from build123d import *

# Parameters (mm, degrees)
SKETCH1_R                  = 3
BOSS_EXTRUDE1_DEPTH        = 15
SHAFT_START                = -15
SHAFT_D_DEPTH              = 15
CUT_EXTRUDE1_DEPTH         = 66.3834841531101
BOSS_EXTRUDE3_DEPTH        = 0.9
CUT_EXTRUDE2_DEPTH         = 59.56795722653927
SHAFT_HOLE_EXPANSION_DEPTH = 59.56795722653927
CUT_EXTRUDE4_DEPTH         = 59.56795722653927
FILLET1_R                  = 2


with BuildPart() as part:
    # Sketch1 → Boss-Extrude1 (new body)
    with BuildSketch(Plane(origin=(0, 0, 0), x_dir=(1, 0, 0), z_dir=(0, 1, 0))):
        with BuildLine():
            Line((-31.81980515339447, 31.819805153394796), (-7.071067811865444, 7.071067811865506))
            ThreePointArc((-7.071067811865444, 7.071067811865506), (4.724e-14, 10.000000000000002), (7.071067811865511, 7.071067811865442))
            Line((7.071067811865511, 7.071067811865442), (31.819805153394796, 31.819805153394476))
            ThreePointArc((31.819805153394796, 31.819805153394476), (-2.4807e-13, -44.99999999999999), (-31.81980515339447, 31.819805153394796))
        make_face()
        with Locations(Location((0, 0, 0), (0, 0, 270))):
            Circle(SKETCH1_R, mode=Mode.SUBTRACT)
    extrude(amount=BOSS_EXTRUDE1_DEPTH)

    # Sketch2 → Shaft D (add)
    with BuildSketch(Plane(origin=(0, 15, 0), x_dir=(1, 0, 0), z_dir=(0, 1, 0)).offset(SHAFT_START)):
        with BuildLine():
            Line((2.499999999999999, 1.6583123951777017), (2.499999999999999, -1.6583123951777017))
            ThreePointArc((2.499999999999999, -1.6583123951777017), (3.0000000000000004, 0), (2.499999999999999, 1.6583123951777017))
        make_face()
    extrude(amount=SHAFT_D_DEPTH)

    # Sketch4 → Cut-Extrude1 (cut, through all)
    with BuildSketch(Plane(origin=(0, 15, 0), x_dir=(1, 0, 0), z_dir=(0, 1, 0))):
        with BuildLine():
            Line((11.490666646784653, -9.641814145298108), (45.50378986806941, 30.893447649017453))
            ThreePointArc((45.50378986806941, 30.893447649017453), (34.99275019793601, -42.43238661193652), (-38.99293957205545, -38.78853778540811))
            Line((-38.99293957205545, -38.78853778540811), (11.490666646784653, -9.641814145298108))
        make_face()
    extrude(amount=-CUT_EXTRUDE1_DEPTH, mode=Mode.SUBTRACT)

    # Sketch6 → Boss-Extrude3 (add)
    with BuildSketch(Plane(origin=(7.0476946558942295, 0, 12.206965220240622), x_dir=(0.8660254037844414, 0, -0.4999999999999952), z_dir=(0.4999999999999952, 0, 0.8660254037844414))):
        Polygon((-42.73546536717619, 15), (5.130302149885087, 15), (5.130302149885089, 0), (-42.73546536717619, 0), align=None)
    extrude(amount=BOSS_EXTRUDE3_DEPTH)

    # Sketch7 → Cut-Extrude2 (cut, through all)
    with BuildSketch(Plane(origin=(0, 15, 0), x_dir=(1, 0, 0), z_dir=(0, 1, 0))):
        with BuildLine():
            Line((-31.525106333140414, 17.38297070940953), (-7.071067811865441, -7.07106781186544))
            Line((-7.071067811865441, -7.07106781186544), (-29.802141727564482, -20.19485945606356))
            ThreePointArc((-29.802141727564482, -20.19485945606356), (-35.962218628181056, -1.6488879097460596), (-31.525106333140414, 17.38297070940953))
        make_face()
    extrude(amount=-CUT_EXTRUDE2_DEPTH, mode=Mode.SUBTRACT)

    # Sketch9 → Shaft Hole Expansion (cut, through all)
    with BuildSketch(Plane(origin=(0, 15, 0), x_dir=(1, 0, 0), z_dir=(0, 1, 0))):
        with BuildLine():
            Line((2.5899999999999985, 1.685229954635274), (2.5899999999999985, -1.6852299546352736))
            ThreePointArc((2.5899999999999985, -1.6852299546352736), (-3.09, 3.8e-16), (2.5899999999999985, 1.685229954635274))
        make_face()
    extrude(amount=-SHAFT_HOLE_EXPANSION_DEPTH, mode=Mode.SUBTRACT)

    # Sketch10 → Cut-Extrude4 (cut, through all)
    with BuildSketch(Plane(origin=(0, 15, 0), x_dir=(1, 0, 0), z_dir=(0, 1, 0))):
        Polygon((11.49066664678465, -9.641814145298104), (7.493411323151681, -14.405557537754012), (21.666837443070385, -15.28946640390601), align=None)
    extrude(amount=-CUT_EXTRUDE4_DEPTH, mode=Mode.SUBTRACT)

    # Fillet1
    # the kernel refuses this fillet: 2 mm, written as the material it adds along each edge
    with BuildSketch(Plane(origin=(-29.802141727564482, 15, 20.19485945606356), x_dir=(0.8660254037844384, 0, -0.5000000000000004), z_dir=(0, -1, 0))) as fillet1_piece_1:
        with BuildLine():
            CenterArc((1.9119296968147805, -2.000000000000001), FILLET1_R, 90.00000000000006, 89.00874965826159)
            ThreePointArc((-0.08777100050710222, -1.9654005617043746), (-0.05731387291771985, -0.9821005956140282), (0, 0))
            Line((0, 0), (1.911929696814779, 4e-17))
        make_face()
    extrude(amount=15)
    with BuildSketch(Plane(origin=(-31.525106333140414, 15, -17.382970709409527), x_dir=(-0.44779859611608247, 0, 0.8941344514760997), z_dir=(0, -1, 0))) as fillet1_piece_2:
        with BuildLine():
            CenterArc((2.77241732034655, -1.9984307521616007), FILLET1_R, 87.73015185982399, 110.66731649351249)
            Line((0.8746374046450249, -2.6296449721851296), (0, 0))
            ThreePointArc((0, 0), (1.4258146218925176, 0.02824646109120102), (2.8516292437850255, 6e-17))
        make_face()
    extrude(amount=15)
    with BuildSketch(Plane(origin=(-7.071067811865441, 15, 7.07106781186544), x_dir=(-0.8660254037844387, 0, 0.4999999999999999), z_dir=(0, -1, 0))) as fillet1_piece_3:
        with BuildLine():
            CenterArc((FILLET1_R * 1.30322537284, FILLET1_R), FILLET1_R, 165.00000000000003, 104.99999999999997)
            Line((FILLET1_R * 0.337299546552, FILLET1_R * 1.2588190451), (0, 0))
            Line((0, 0), (FILLET1_R * 1.30322537284, 1e-17))
        make_face()
    extrude(amount=15)
    with BuildSketch(Plane(origin=(-7.071067811865445, 0, -7.071067811865506), x_dir=(-0.7071067811865437, 0, -0.7071067811865515), z_dir=(0, 1, 0))) as fillet1_piece_4:
        with BuildLine():
            CenterArc((1.8321595661992367, -2), FILLET1_R, 89.99999999999999, 80.40593177313956)
            ThreePointArc((-0.13986702816730157, -1.666666666666667), (-0.0350281054503974, -0.8362626027968331), (0, 0))
            Line((0, 0), (1.8321595661992371, 5e-17))
        make_face()
    extrude(amount=15)
    with BuildSketch(Plane(origin=(7.071067811865512, 0, -7.071067811865442), x_dir=(0.7071067811865507, 0, -0.7071067811865444), z_dir=(0, 1, 0))) as fillet1_piece_5:
        with BuildLine():
            CenterArc((1.8321595661992343, 2.0000000000000004), FILLET1_R, 189.59406822686037, 80.40593177313957)
            ThreePointArc((-0.139867028167305, 1.6666666666666698), (-0.03502810545039883, 0.8362626027968333), (0, 0))
            Line((0, 0), (1.8321595661992325, 4e-17))
        make_face()
    extrude(amount=15)
    # the kernel refuses this fillet: 2 mm, written as the material it takes off along each edge
    with BuildSketch(Plane(origin=(-29.512303994630546, -4.175823272127531, 34.35412076723451), x_dir=(-0.49999999999865496, 0, -0.8660254037852152), z_dir=(0, 1, 0))) as fillet1_2_piece_1:
        with BuildLine():
            CenterArc((2.0000000000025833, -1.6703293088479174), FILLET1_R, 123.36701296928852, 56.63298703080011)
            Line((2.58454e-12, -1.6703293088510118), (0, 0))
            Line((0, 0), (0.9000000000009275, 2e-17))
        make_face()
    extrude(amount=23.35164654425506, mode=Mode.SUBTRACT)
    with BuildSketch(Plane(origin=(9.799219929370043, -0.8816349035423467, 11.657601847458647), x_dir=(0.6427876096865316, 0, -0.7660444431189845), z_dir=(0, 1, 0))) as fillet1_2_piece_2:
        with BuildLine():
            CenterArc((FILLET1_R * 0.176326980708, FILLET1_R), FILLET1_R, 249.99999999999906, 20.000000000000284)
            Line((-FILLET1_R * 0.165693162617, FILLET1_R * 0.0603073792141), (0, 0))
            Line((0, 0), (FILLET1_R * 0.176326980708, 1e-17))
        make_face()
    extrude(amount=16.763269807084693, mode=Mode.SUBTRACT)
    with BuildSketch(Plane(origin=(38.76183530710732, 18.67919870008775, -22.858699079883973), x_dir=(-0.5219883581091025, 0, -0.8529526094681715), z_dir=(0, -1, 0))) as fillet1_2_piece_3:
        with BuildLine():
            CenterArc((1.4389754915898811, -1.9997325944085071), FILLET1_R, 89.06305798679442, 72.40266339187922)
            Line((-0.45729180864609936, -1.363988678939587), (0, 0))
            ThreePointArc((0, 0), (0.7358397400175548, 0.00601662580861232), (1.4716794800350999, 0))
        make_face()
    extrude(amount=22.3583974001755, mode=Mode.SUBTRACT)


solid = part.part
Check sheet for the modelled part. Datum: model origin and axes. Units: mm. A direction names the side the tool comes from. Round coordinates to 2 decimals unless told otherwise and drop trailing zeros. Write each loop counter-clockwise with the first axis right and the second up, starting at its lowest first coordinate (ties: lowest second). Pieces come first, ordered by that corner, then holes. Notation, with made-up numbers: (-7.75, 76.5) -> (9.25, 76.5) arc R9 ccw to (9.25, 92.5) -> close; hole circle Ø6 at (-21.5, 0). An arc over 180 degrees is marked (long way). Answer as CSV lines item,"result". Start each with the question number.
1) Tool access check on faces 1 (the flat face through (-20, 7, -20)), 2 (the cylindrical face through (38.3, 7.6, -22.9)), 3 (the cylindrical face through (-29.626, 7.605, 19.448)). Record the directions out of +Z, -Z, +X, -X, +Y, -Y that give a thin tool (end or side, any length) a straight path to the whole face; none if there is none.
2) Release check for a two-part mould opening along Z. For faces 4 (the cylindrical face through (-29.021, 7.395, 33.786)), 5 (the flat face through (-18.606, 7.605, 13.731)), 6 (the cylindrical face through (35.075, 7.395, -28.191)) record: pulls with the +Z half, pulls with the -Z half, needs draft (parallel to the pull), parting line crosses it, or undercut.
3) Section check B-B on z = 0. Enter the section's corners in (x, y), and give its area (3 significant figures).
4) Section check A-A on y = 5.25. Enter the section's corners in (x, z), and give its area (3 significant figures).
5) Go/stop test with flat-tipped pins: P1, Ø6, axis at y = 7.5, z = 25.5, coming from the +X side; P2, Ø8, axis at y = 2, z = 19.5, coming from the +X side; P3, Ø4, axis at x = -2.5, y = 4.5, coming from the -Z side; P4, Ø5, axis at x = 0, z = 0, coming from the -Y side. Record where each tip stops, or that it passes through.
6) Section check C-C on x = -18. Enter the section's corners in (y, z), and give its area (3 significant figures).
7) Section check D-D on x = 0. Enter the section's corners in (y, z), and give its area (3 significant figures).
8) Material ranges on line 1 (X direction, y = 9.5, z = 2.5); line 2 (X direction, y = 12.5, z = -15); line 3 (X direction, y = 4.25, z = -18), recorded low to high. Write a range as from..to.
Found:
1,face 1,"-Z, +Y, -Y"
1,face 2,"+X, +Y, -Y"
1,face 3,"+Y, -Y"
2,face 4,"pulls with the +Z half"
2,face 5,"undercut"
2,face 6,"pulls with the -Z half"
3,outline,"(-45, 0) -> (-36, 0) -> (-36, 15) -> (-45, 15) -> close; (-14.14, 0) -> (-3.09, 0) -> (-3.09, 15) -> (-14.14, 15) -> close; (2.59, 0) -> (19.58, 0) -> (19.58, 15) -> (2.59, 15) -> close"
3,area,"556 mm^2"
4,outline,"(-31.82, -31.82) -> (-8.37, -8.37) arc R2 cw to (-5.79, -8.15) arc R10 ccw to (5.79, -8.15) arc R2 cw to (8.37, -8.37) -> (31.82, -31.82) arc R45 ccw to (37.99, -24.11) arc R2 ccw to (37.84, -21.76) -> (10.03, 11.39) arc R2 ccw to (9.49, 11.83) -> (-28.07, 33.52) arc R2 ccw to (-29.96, 33.57) arc R45 ccw to start; hole (-32.8, -14.83) arc R2 ccw to (-29.57, -15.42) -> (-8.91, 5.23) arc R2 ccw to (-9.33, 8.37) -> (-28.15, 19.24) arc R2 ccw to (-30.86, 18.54) arc R36 ccw to start; hole (2.59, -1.69) -> (2.59, 1.69) arc R3.09 ccw (long way) to start"
4,area,"2,080 mm^2"
5,P1,"stops at x = -8.98"
5,P2,"stops at x = 3.14"
5,P3,"stops at z = -9.99"
5,P4,"passes through"
6,outline,"(0, -18) -> (15, -18) -> (15, -3.86) -> (0, -3.86) -> close; (0, 13.38) -> (15, 13.38) -> (15, 27.71) -> (0, 27.71) -> close"
6,area,"427 mm^2"
7,outline,"(0, -10) -> (15, -10) -> (15, -3.09) -> (0, -3.09) -> close; (0, 3.09) -> (15, 3.09) -> (15, 17.32) -> (0, 17.32) -> close"
7,area,"317 mm^2"
8,line 1,"x = -44.93..-35.91, -11.64..-1.82, 1.82..17.48"
8,line 2,"x = -42.43..-32.72, -29.14..-15, 15..32.17"
8,line 3,"x = -41.24..-18, 18..34.68"
